Source: CAD feature listing. Evaluate the final solid. Frame: model axes, mm. A direction names the side the tool comes from. Give positions to 0.01 mm unless a question says otherwise; leave off trailing zeros. Order: outer loops, then holes, each group sorted by start corner. A loop starts at its lowest first (then second) coordinate and runs counter-clockwise, first axis right, second up. Notation, with made-up numbers: M -20,49.5 L 28,49.5 A8 cw 28,57.5 Z; hole C 59.25,-2 d4. An arc over 180 degrees is marked long. Use CSV: the item, a comma, the result in double quotes. Start each with the question number.
Item 1: Section query A-A on x = 0. Return loops of the section in (y, z) (3 decimals), and give its area (3 significant figures).
Item 2: Section query D-D on y = 18. Return loops of the section in (x, z), and give its area (3 significant figures).
Item 3: Section query C-C on y = 0. Return loops of the section in (x, z) (3 decimals), and give its area (3 significant figures).
Item 4: Ray query, probe 1 along X at (y, z) = (0, 22.5) (3 decimals); probe 2 along Y at (x, z) = (0, 15) (3 decimals); probe 3 along Z at (x, y) = (3, 36). Return the intervals inside material, ascending. Write a range as from..to.
Item 5: Access query for faces 1 (the face through (1.24, 63.589, 47.544)), 2 (the face through (2.64, -4.02, 58.24)), 3 (the face through (-4.8, 21.7, 14.5)). Directions: +Z, -Z, +X, -X, +Y, -Y. A direction counts if a zero-diameter tool reaches every point of the face in a straight line with its end or side. Return the directions, or none.
Item 6: Pull-direction query (Y, two-part tool) for faces 4 (the face through (36.29, 67.94, 38.54)), 5 (the face through (21, 15, 0)), 6 (the face through (0, -63.5, 39)); classes: +Y half, -Y half, draft (parallel to the pull), parting line (faces both ways), or undercut.
Item 7: First-contact query: pin 1 (5.5 mm diameter, centred on x = 18.5, y = 8.5, fed in from -Z). Flat tip, straight axial feed; report the tip coordinate or a pass-through.
Item 8: Section query B-B on y = -54. Return loops of the section in (x, z), and give its area (3 significant figures).
from build123d import *

# Parameters (mm, degrees)
F0_W      = 76.2
F0_H      = 139.7
F1_DEPTH  = 76.2
F3_R      = 6.35
F2_R      = 22.225
F4_DEPTH  = 12.7
F6_R      = 9.525
F7_DEPTH  = 12.7
F8_R      = 9.525
F9_DEPTH  = 120.65
F9_TAPER  = -10
F5_R      = 22.225
F10_DEPTH = 25.4


with BuildPart() as f1:
    # F0 (on Top) → F1 (new body)
    with BuildSketch(Plane.XY):
        Rectangle(F0_W, F0_H)
    extrude(amount=F1_DEPTH)

    # F3
    f3_edges = [f1.edges().sort_by_distance(p)[0] for p in [
        (38.1, 0, 76.2),
        (0, 69.85, 76.2),
        (-38.1, 0, 76.2),
        (0, -69.85, 76.2),
        (38.1, 69.85, 38.1),
        (-38.1, 69.85, 38.1),
        (0, 69.85, 0),
        (38.1, -69.85, 38.1),
        (38.1, 0, 0),
        (0, -69.85, 0),
        (-38.1, -69.85, 38.1),
        (-38.1, 0, 0),
    ]]
    fillet(f3_edges, radius=F3_R)

    # F2 (on face) → F4 (cut)
    with BuildSketch(Plane(origin=(0, 0, 0), x_dir=(1, 0, 0), z_dir=(0, 0, -1))):
        Circle(F2_R)
    extrude(amount=-F4_DEPTH, mode=Mode.SUBTRACT)

    # F6 (on face) → F7 (cut)
    with BuildSketch(Plane(origin=(0, 69.85, 0), x_dir=(-1, 0, 0), z_dir=(0, 1, 0))):
        with Locations((0, 38.1)):
            Circle(F6_R)
    extrude(amount=-F7_DEPTH, mode=Mode.SUBTRACT)

    # F8 (on face) → F9 (cut)
    with BuildSketch(Plane(origin=(0, 57.15, 0), x_dir=(-1, 0, 0), z_dir=(0, 1, 0))):
        with Locations((0, 38.1)):
            Circle(F8_R)
    extrude(amount=-F9_DEPTH, taper=F9_TAPER, mode=Mode.SUBTRACT)

    # F5 (on face) → F10 (cut)
    with BuildSketch(Plane(origin=(0, 0, 12.7), x_dir=(1, 0, 0), z_dir=(0, 0, -1))):
        Circle(F5_R)
    extrude(amount=-F10_DEPTH, mode=Mode.SUBTRACT)


solid = f1.part
Verdict:
1,outline,"M -69.85,6.35 A6.35 ccw -63.5,0 L -22.225,0 L -22.225,14.579 L -63.5,7.301 L -63.5,68.899 L 57.15,47.625 L 69.85,47.625 L 69.85,69.85 A6.35 ccw 63.5,76.2 L -63.5,76.2 A6.35 ccw -69.85,69.85 Z; M 22.225,0 L 63.5,0 A6.35 ccw 69.85,6.35 L 69.85,28.575 L 57.15,28.575 L 22.225,22.417 Z"
1,area,"4,680 mm2"
2,outline,"M -38.1,6.35 A6.35 ccw -31.75,0 L -13.04,0 L -13.04,28.1 A16.43 cw long 13.04,28.1 L 13.04,0 L 31.75,0 A6.35 ccw 38.1,6.35 L 38.1,69.85 A6.35 ccw 31.75,76.2 L -31.75,76.2 A6.35 ccw -38.1,69.85 Z"
2,area,"4,310 mm2"
3,outline,"M -38.1,6.35 A6.35 ccw -31.75,0 L -22.225,0 L -22.225,38.1 L -19.602,38.1 A19.602 cw 19.602,38.1 L 22.225,38.1 L 22.225,0 L 31.75,0 A6.35 ccw 38.1,6.35 L 38.1,69.85 A6.35 ccw 31.75,76.2 L -31.75,76.2 A6.35 ccw -38.1,69.85 Z"
3,area,"3,470 mm2"
4,probe 1,"-38.1..-22.225, 22.225..38.1"
4,probe 2,"-69.85..-63.5, 22.225..69.85"
4,probe 3,"0..25.19, 51.01..76.2"
5,face 1,"+Y"
5,face 2,"none"
5,face 3,"-Z"
6,face 4,"+Y half"
6,face 5,"draft"
6,face 6,"undercut"
7,pin 1,"z = 0"
8,outline,"M -38.1,6.35 A6.35 ccw -31.75,0 L 31.75,0 A6.35 ccw 38.1,6.35 L 38.1,69.85 A6.35 ccw 31.75,76.2 L -31.75,76.2 A6.35 ccw -38.1,69.85 Z; hole C 0,38.1 d58.25"
8,area,"3,110 mm2"
